Design review of the part built by this model. Coordinates are the model's own, in mm. Face numbers are marked on the shaded views. Give positions to 0.01 mm unless a question says otherwise; leave off trailing zeros. Loops run counter-clockwise (first coordinate to the right, second up) from the corner with the lowest first, then second, coordinate; pieces in that order, holes last.
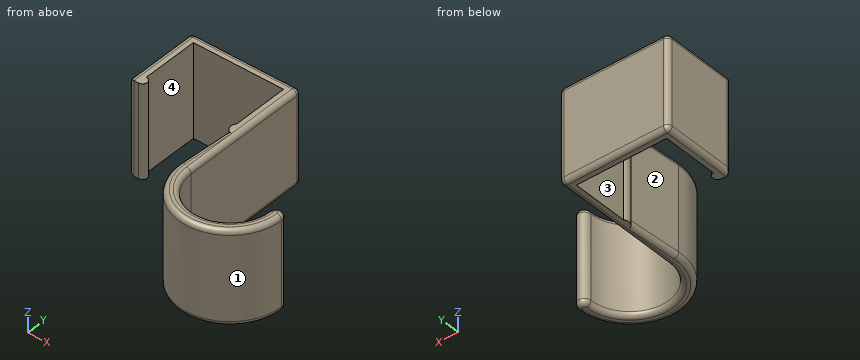
Autodesk Fusion 360 part; units mm, degrees
sketch "Sketch1" plane through (0, 0, 0) normal (0, 0, 1) x (1, 0, 0)
  line L0 (14.5, 9) -> (-14.5, 9)
  line L1 (-14.5, 9) -> (-14.5, -9)
  line L2 (14.5, -9) -> (14.5, 9)
  line L3 (14.5, 9) -> (-14.5, -9) construction
  line L4 (-14.5, 9) -> (14.5, -9) construction
  line L5 (17.5, -12) -> (17.5, 12)
  line L6 (17.5, 12) -> (-17.5, 12)
  line L7 (-17.5, 12) -> (-17.5, -12)
  arc A0 (14.5, -9) -> (14.5, -12) centre (16.25, -10.5) ccw
  arc A1 (-14.5, -12) -> (-14.5, -9) centre (-14.5, -10.5) ccw
  line L8 (-17.5, -12) -> (-14.5, -12)
  line L9 (17.5, -12) -> (17.5, -30)
  line L10 (14.5, -12) -> (13.5268, -29.0603)
  arc A2 (17.5, -29.9983) -> (42.5, -30) centre (30, -30) ccw
  arc A3 (13.5268, -29.0603) -> (46.5, -30) centre (30, -30) ccw
  arc A4 (46.5, -30) -> (42.5, -30) centre (44.5, -29.8577) ccw
  dimension "d1" = 29
  dimension "d2" = 18
  dimension "d4" = 25
  dimension "d5" = 33
extrude "Extrude1" add sketch "Sketch1" along normal blind 30
fillet "Fillet1" radius 1.5 5 edges at (29.9991, -42.5, 30) (17.5, -8.9991, 30) (44.5, -27.8527, 30) (14.0134, -20.5301, 30) (29.5299, -46.4933, 30)
fillet "Fillet2" radius 1.5 5 edges at (17.5, -8.9991, 0) (29.9991, -42.5, 0) (44.5, -27.8527, 0) (14.0134, -20.5301, 0) (29.5299, -46.4933, 0)
fillet "Fillet3" radius 1.5 5 edges at (-0.75, 12, 0) (17.0607, 12, 0.4393) (17.5, 12, 15) (17.0607, 12, 29.5607) (-0.75, 12, 30)
fillet "Fillet4" radius 1.5 1 faces at (-17.5, -4, 19.5)
Q1. Insertion check: pin 1 (12 mm diameter, centred on x = 36, y = -25.5, fed in from -Z); pin 2 (14.5 mm diameter, centred on y = 0.5, z = 20, fed in from +X); pin 3 (0.8 mm diameter, centred on x = -15.5, z = 18.5, fed in from -Y); pin 4 (1 mm diameter, centred on x = 20, z = 9.5, fed in from +Y). Each pin has a flat end and moves straight along its axis. Give the tip position at first contact, or say it passes through.
Results:
pin 1: passes through
pin 2: stops at x = 17.5
pin 3: stops at y = -12
pin 4: stops at y = -36.78
Q2. Wall thickness on line 1 (X direction, y = 0.5, z = 6); line 2 (Y direction, x = -8, z = 23); line 3 (Y direction, x = 30.5, z = 11.5): over which ranges is each line inside the solid? List them lowest first.
Results:
line 1: x = -17.5 to -14.5, 14.5 to 17.5
line 2: y = 9 to 12
line 3: y = -46.49 to -42.49
Q3. Draft analysis for pull direction X (two halves, no side actions). For the marked faces 1, 2, 3 and 4, state which applies: pulls with the +X half, pulls with the -X half, needs draft (parallel to the pull), parting line crosses it, or undercut.
Results:
face 1: parting line crosses it
face 2: pulls with the -X half
face 3: undercut
face 4: undercut
Q4. Take a section at C-C (x = -5.5). Give the boundary of the cut face in (y, z), plus the area to 3 significant figures.
Results:
outline: (9, 0) - (10.5, 0) arc R1.5 ccw to (12, 1.5) - (12, 28.5) arc R1.5 ccw to (10.5, 30) - (9, 30) - close
area: 89.0 mm2
Q5. Take a section at B-B (z = 22). Give the boundary of the cut face in (x, y), plus the area to 3 significant figures.
Results:
outline: (-17.5, -10.5) arc R1.5 ccw to (-16, -12) - (-14.5, -12) arc R1.5 ccw to (-14.5, -9) - (-14.5, 9) - (14.5, 9) - (14.5, -9) arc R2.3 ccw to (14.5, -12) - (13.53, -29.06) arc R16.5 ccw (long way) to (46.5, -30) arc R2.01 ccw (long way) to (42.5, -30) arc R12.5 cw to (17.5, -30) - (17.5, 10.5) arc R1.5 ccw to (16, 12) - (-16, 12) arc R1.5 ccw to (-17.5, 10.5) - close
area: 487 mm2
Q6. Take a section at A-A (y = 5). Give the boundary of the cut face in (x, z), plus the area to 3 significant figures.
Results:
outline: (-17.5, 1.5) arc R1.5 ccw to (-16, 0) - (-14.5, 0) - (-14.5, 30) - (-16, 30) arc R1.5 ccw to (-17.5, 28.5) - close; (14.5, 0) - (16, 0) arc R1.5 ccw to (17.5, 1.5) - (17.5, 28.5) arc R1.5 ccw to (16, 30) - (14.5, 30) - close
area: 178 mm2
